Input: part model. Units: mm. Frame: model coordinates. Face numbers are marked on the shaded views. A direction names the side the tool comes from. Give positions to 0.01 mm unless a question says otherwise; leave off trailing zeros. Loops run counter-clockwise (first coordinate to the right, second up) from the corner with the lowest first, then second, coordinate; pieces in that order, holes last.
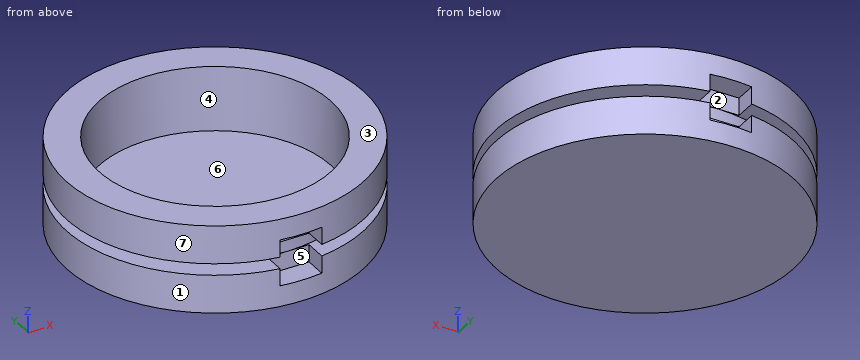
from build123d import *

# Parameters (mm, degrees)
SKETCH7_W          = 9
SKETCH7_H          = 10
CUT_EXTRUDE1_DEPTH = 5


with BuildPart() as part:
    # Sketch2 → Revolve1 (revolve)
    with BuildSketch(Plane(origin=(0, 0, 0), x_dir=(0, 0, -1), z_dir=(1, 0, 0)), mode=Mode.PRIVATE) as revolve1_sk:
        Polygon((0, 0), (0, 32), (-8.25, 32), (-8.25, 27), (-10.75, 27), (-10.75, 32), (-19, 32), (-19, 25), (-5, 25), (-5, 0), align=None)
    revolve(revolve1_sk.sketch.rotate(Axis((0, 0, 5), (0, 0, -1)), 90), axis=Axis((0, 0, 5), (0, 0, -1)))

    # Sketch7 → Cut-Extrude1 (cut)
    with BuildSketch(Plane(origin=(0, 32, 0), x_dir=(1, 0, 0), z_dir=(0, 1, 0))):
        with Locations((0, -9.5)):
            Rectangle(SKETCH7_W, SKETCH7_H)
    cut_extrude1 = extrude(amount=-CUT_EXTRUDE1_DEPTH, mode=Mode.SUBTRACT)

    # Mirror1: Cut-Extrude1 across plane
    add(cut_extrude1.mirror(Plane.ZX), mode=Mode.SUBTRACT)


solid = part.part
(1) Pin query (flat end, axial travel): pin 1 Ø4 at (y, z) = (28.5, 12.5) entering from -X; pin 2 Ø1.9 at (y, z) = (29.5, 13) entering from +X; pin 3 Ø15 at (x, y) = (-10.5, -8.5) entering from +Z. Return the tip coordinate at first contact, or that it passes through.
Values follow:
pin 1: stops at x = -17.94
pin 2: stops at x = 14.45
pin 3: stops at z = 5
(2) Reachability of the marked faces 5, 6 and 7 from +Z, -Z, +X, -X, +Y, -Y: full face, straight path, thin tool, end or side. Return the list, or none.
Values follow:
face 5: -Y
face 6: +Z
face 7: +Z, -Z
(3) Cut plane C-C (x = 16). Return the cut outline in (y, z).
Values follow:
outline: (-27.71, 0) - (27.71, 0) - (27.71, 8.25) - (21.75, 8.25) - (21.75, 10.75) - (27.71, 10.75) - (27.71, 19) - (19.21, 19) - (19.21, 5) - (-19.21, 5) - (-19.21, 19) - (-27.71, 19) - (-27.71, 10.75) - (-21.75, 10.75) - (-21.75, 8.25) - (-27.71, 8.25) - close
(4) Cut plane D-D (x = 26). Return the cut outline in (y, z).
Values follow:
outline: (-18.65, 0) - (18.65, 0) - (18.65, 8.25) - (7.28, 8.25) - (7.28, 10.75) - (18.65, 10.75) - (18.65, 19) - (-18.65, 19) - (-18.65, 10.75) - (-7.28, 10.75) - (-7.28, 8.25) - (-18.65, 8.25) - close
(5) Cut plane B-B (y = 0). Return the cut outline in (x, z).
Values follow:
outline: (-32, 0) - (32, 0) - (32, 8.25) - (27, 8.25) - (27, 10.75) - (32, 10.75) - (32, 19) - (25, 19) - (25, 5) - (-25, 5) - (-25, 19) - (-32, 19) - (-32, 10.75) - (-27, 10.75) - (-27, 8.25) - (-32, 8.25) - close
(6) Cut plane A-A (z = 13.5). Return the cut outline in (x, y), and give its area (3 significant figures).
Values follow:
outline: (-4.5, -31.68) - (-4.5, -27) - (4.5, -27) - (4.5, -31.68) arc R32 ccw to (4.5, 31.68) - (4.5, 27) - (-4.5, 27) - (-4.5, 31.68) arc R32 ccw to start; hole circle Ø50 at (0, 0)
area: 1,170 mm2
(7) Ray query, probe 1 along Y at (x, z) = (0.5, 13) (3 decimals); probe 2 along Z at (x, y) = (-18.5, 13); probe 3 along X at (y, z) = (-28, 5). Return the intervals inside material, ascending.
Values follow:
probe 1: y = -27 to -24.995, 24.995 to 27
probe 2: z = 0 to 5
probe 3: x = -15.49 to -4.5, 4.5 to 15.49
(8) Mould query, pull axis X, two halves, no side actions, for the marked faces 1, 2, 3 and 4. Classes: +X half, -X half, draft (parallel to the pull), parting line (faces both ways), or undercut.
Values follow:
face 1: parting line
face 2: undercut
face 3: draft
face 4: undercut
